Verification items for the finished model (mm, model axes). Coordinates: 2 decimals unless noted, no trailing zeros. Write each loop counter-clockwise with the first axis right and the second up, starting at its lowest first coordinate (ties: lowest second). Pieces come first, ordered by that corner, then holes. Notation, with made-up numbers: (40.5, 64.5) -> (61.5, 64.5) arc R14 cw to (61.5, 83.5) -> close; hole circle Ø2 at (-16, 11.5). An arc over 180 degrees is marked (long way). Write item = value, one per line. Start each with the question number.
(1) Section check A-A (y = 2.85). Record the cut outline in (x, z).
(2) Section check B-B (z = 809). Record the cut outline in (x, y), plus the area to 4 significant figures.
(3) Gauge pin test, flat ends, axial feed: pin 1 Ø3.5 at (x, z) = (139.1, 731.75) entering from +Y; pin 2 Ø1.5 at (x, y) = (-297.5, 3.5) entering from +Z. Record the tip position at first contact, or that the pin passes through.
(4) Material ranges on probe 1 along X at (y, z) = (3.75, 708); probe 2 along X at (y, z) = (3.15, 736); probe 3 along X at (y, z) = (3.9, 776), recorded low to high. Write a range as [from, to].
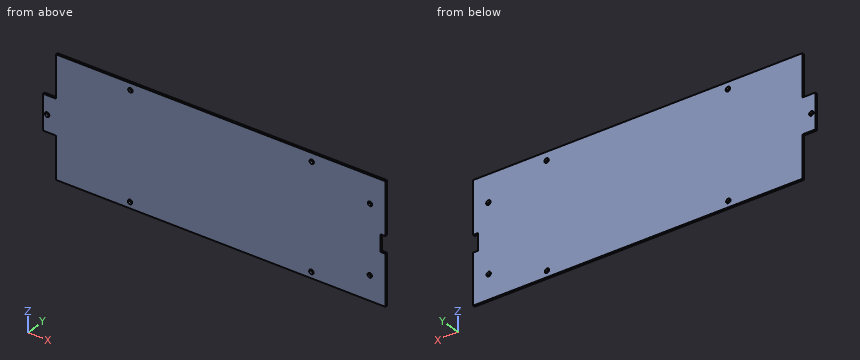
```python
from build123d import *

# Parameters (mm, degrees)
BOSS_EXTRUDE1_START = 2
SKETCH1_R           = 3
SKETCH1_R_2         = 3.000000004
SKETCH1_R_3         = 2.999999993
BOSS_EXTRUDE1_DEPTH = 3


with BuildPart() as part:
    # Sketch1 → Boss-Extrude1 (new body)
    with BuildSketch(Plane(origin=(0, 0, 0), x_dir=(1, 0, 0), z_dir=(0, 1, 0)).offset(BOSS_EXTRUDE1_START)):
        Polygon((-302.235528935, -755.752958265), (-284.735528935, -755.752958265), (-284.735528935, -699.252958265), (160.264471065, -699.252958265), (160.264471065, -766.790866852), (153.764471065, -766.790866852), (153.764471065, -789.390866852), (160.264471065, -789.390866852), (160.264471065, -859.252958265), (-284.735528935, -859.252958265), (-284.735528935, -802.752958265), (-302.235528935, -802.752958265), align=None)
        with Locations(Location((-296.74646616, -778.09086684, 0), (0, 0, 270))):
            Circle(SKETCH1_R, mode=Mode.SUBTRACT)
        with Locations(Location((139.102370463, -731.752958265, 0), (0, 0, 270))):
            Circle(SKETCH1_R_2, mode=Mode.SUBTRACT)
        with Locations(Location((139.486711965, -823.034841954, 0), (0, 0, 270))):
            Circle(SKETCH1_R, mode=Mode.SUBTRACT)
        with Locations(Location((-184.735528935, -707.46118256, 0), (0, 0, 270))):
            Circle(SKETCH1_R_2, mode=Mode.SUBTRACT)
        with Locations(Location((60.264471065, -707.46118256, 0), (0, 0, 270))):
            Circle(SKETCH1_R_2, mode=Mode.SUBTRACT)
        with Locations(Location((60.856164784, -847.989637054, 0), (0, 0, 270))):
            Circle(SKETCH1_R, mode=Mode.SUBTRACT)
        with Locations(Location((-184.135148537, -850.052740812, 0), (0, 0, 270))):
            Circle(SKETCH1_R_3, mode=Mode.SUBTRACT)
    extrude(amount=BOSS_EXTRUDE1_DEPTH)


solid = part.part
```
Response:
q1.outline = (-302.24, 755.75) -> (-284.74, 755.75) -> (-284.74, 699.25) -> (160.26, 699.25) -> (160.26, 766.79) -> (153.76, 766.79) -> (153.76, 789.39) -> (160.26, 789.39) -> (160.26, 859.25) -> (-284.74, 859.25) -> (-284.74, 802.75) -> (-302.24, 802.75) -> close; hole circle Ø6 at (-296.75, 778.09); hole circle Ø6 at (-184.74, 707.46); hole circle Ø6 at (-184.14, 850.05); hole circle Ø6 at (60.26, 707.46); hole circle Ø6 at (60.86, 847.99); hole circle Ø6 at (139.1, 731.75); hole circle Ø6 at (139.49, 823.03)
q2.outline = (-284.74, 2) -> (160.26, 2) -> (160.26, 5) -> (-284.74, 5) -> close
q2.area = 1,335 mm2
q3.pin_1 = through
q3.pin_2 = 802.75
q4.probe_1 = [-284.74, -187.69], [-181.78, 57.31], [63.22, 160.26]
q4.probe_2 = [-284.74, 160.26]
q4.probe_3 = [-302.24, -298.9], [-294.6, 153.76]
